Verification items for the finished model (mm, model axes). A direction names the side the tool comes from. Round coordinates to 2 decimals unless told otherwise and drop trailing zeros. Write each loop counter-clockwise with the first axis right and the second up, starting at its lowest first coordinate (ties: lowest second). Pieces come first, ordered by that corner, then holes. Notation, with made-up numbers: M 46.5,73.5 L 57.5,73.5 A25 ccw 57.5,89.5 Z; hole C 56.25,87 d7. An arc over 180 degrees is marked long. One line per item, written item: value. Start each with the question number.
Item 1: Section check A-A, the plane z = -27. Record the cut outline in (x, y), then the cut area to 3 significant figures.
Item 2: Draft check along Y on faces 1 (the face through (-3.7, -24.2, -2.4)), 2 (the face through (-36, -17, -31)), 3 (the face through (-47, -17, -31)), 4 (the face through (28, -4, 0)). Enter one of: +Y half, -Y half, draft (parallel to the pull), parting line (faces both ways), or undercut.
Item 3: Section check B-B, the plane x = -10. Record the cut outline in (y, z), then the cut area to 3 significant figures.
Item 4: Section check C-C, the plane y = -21. Record the cut outline in (x, z).
Item 5: Thickness scan on probe 1 along Z at (x, y) = (14, -3); probe 2 along Y at (x, z) = (-30, 32); probe 3 along Z at (x, y) = (-21, -4). Record the ranges inside material, lowest first. Write a range as from..to.
Item 6: Tool access check on faces 5 (the face through (0, -15, -1)), 6 (the face through (-23, -17, 24)), 7 (the face through (-21, -17, 38)). Record the directions out of +Z, -Z, +X, -X, +Y, -Y that give a thin tool (end or side, any length) a straight path to the whole face; none if there is none.
Item 7: Gauge pin test, flat ends, axial feed: pin 1 (5 mm diameter, centred on x = 18, z = 5, fed in from -Y); pin 2 (10.5 mm diameter, centred on y = -21, z = 0, fed in from -X); pin 3 (12 mm diameter, centred on y = -29.5, z = 29.5, fed in from +X). Record the tip position at first contact, or that the pin passes through.
Item 8: Section check D-D, the plane y = -14. Record the cut outline in (x, z), then the cut area to 3 significant figures.
Autodesk Fusion 360 part; units mm, degrees
sketch "Sketch1" plane through (0, 0, 0) normal (0, 0, 1) x (1, 0, 0)
  line L0 (0, 0) -> (-30, 0)
  line L1 (-30, -34) -> (0, -34)
  line L2 (0, -34) -> (0, 0)
  line L3 (0, 0) -> (28, 0)
  line L4 (28, 0) -> (28, -8)
  line L5 (28, -8) -> (0, -8)
  line L6 (0, -8) -> (0, 0)
  arc A0 (-30, 0) -> (-30, -34) centre (-30, -17) ccw
  circle A1 centre (-30, -17) radius 6
  line L7 (-7.5, 0) -> (-7.5, -34)
  dimension "d2" = 28
  dimension "d3" = 8
  dimension "d4" = 34
  dimension "d5" = 34
  dimension "d6" = 17
  dimension "d7" = 12
  dimension "d8" = 30
  dimension "d9" = 7.5
sketch "Sketch2" plane through (0, 0, 0) normal (0, 1, 0) x (1, 0, 0)
  circle A0 centre (14, -27) radius 4
  line L0 (20, -38) -> (28, -38)
  line L1 (28, -38) -> (28, -30)
  arc A1 (20, -38) -> (28, -30) centre (20, -30) ccw
  dimension "d18" = 8
  dimension "d19" = 27
  dimension "d20" = 14
  dimension "d29" = 16
  dimension "d30" = 38
  dimension "d31" = 28
sketch "Sketch3" plane through (0, 0, 0) normal (1, 0, 0) x (0, 1, 0)
  circle A0 centre (-21, 0) radius 4
  line L0 (0, 0) -> (-21, 0) construction
  dimension "d22" = 8
  dimension "d23" = 21
extrude "Extrude1" add sketch "Sketch1" along normal blind 38 and the other way blind 38
extrude "Extrude2" cut sketch "Sketch1" along normal blind 24 and the other way blind 24 contours L0 L1 A0 L7
extrude "Extrude3" cut sketch "Sketch2" against normal through all
extrude "Extrude4" cut sketch "Sketch3" against normal through all
mirror "Mirror1" about plane through (0, 0, 0) normal (0, 0, 1) of "Extrude3"
equation "d4 = ( 17 * 2 ) * 1 mm"
equation "d5 = ( 17 * 2 ) * 1 mm"
equation "d10 = ( 76 / 2 ) * 1 mm"
equation "d12 = ( 76 / 2 ) * 1 mm"
equation "d14 = ( 76 / 2 ) * 1 mm - 14 mm"
equation "d16 = ( 76 / 2 ) * 1 mm - 14 mm"
equation "d19 = ( 76 / 2 ) * 1 mm - 11 mm"
equation "d23 = ( 17 * 2 ) * 1 mm - 13 mm"
equation "d30 = ( 76 / 2 ) * 1 mm"
Response values:
1. outline: M -30,-34 L 0,-34 L 0,-8 L 10,-8 L 10,0 L -30,0 A17 ccw Z; M 18,-8 L 28,-8 L 28,0 L 18,0 Z; hole C -30,-17 d12
1. area: 1,520 mm2
2. face 1: undercut
2. face 2: undercut
2. face 3: parting line
2. face 4: draft
3. outline: M -34,-38 L 0,-38 L 0,-24 L -34,-24 Z; M -34,24 L 0,24 L 0,38 L -34,38 Z
3. area: 952 mm2
4. outline: M -46.52,-38 L -34.47,-38 L -34.47,-24 L -46.52,-24 Z; M -46.52,24 L -34.47,24 L -34.47,38 L -46.52,38 Z; M -25.53,-38 L 0,-38 L 0,-4 L -7.5,-4 L -7.5,-24 L -25.53,-24 Z; M -25.53,24 L -7.5,24 L -7.5,4 L 0,4 L 0,38 L -25.53,38 Z
5. probe 1: z = -38..-31, -23..23, 31..38
5. probe 2: y = -34..-23, -11..0
5. probe 3: z = -38..-24, 24..38
6. face 5: +Z, -Z, +X, -Y
6. face 6: -X, +Y, -Y
6. face 7: +Z, +X, -X, +Y, -Y
7. pin 1: stops at y = -8
7. pin 2: stops at x = -7.5
7. pin 3: stops at x = 0
8. outline: M -46.73,-38 L -35.2,-38 L -35.2,-24 L -46.73,-24 Z; M -46.73,24 L -35.2,24 L -35.2,38 L -46.73,38 Z; M -24.8,-38 L 0,-38 L 0,38 L -24.8,38 L -24.8,24 L -7.5,24 L -7.5,-24 L -24.8,-24 Z
8. area: 1,380 mm2
